from build123d import *

# Parameters (mm, degrees)
BOSS_EXTRUDE1_DEPTH = 6.5
SCALE1_SCALE        = 0.85
SKETCH2_R           = 9
CUT_EXTRUDE1_DEPTH  = 10
SKETCH7_R           = 2.1
CUT_EXTRUDE7_DEPTH  = 6
SKETCH8_R           = 2.1
CUT_EXTRUDE8_DEPTH  = 6
SKETCH9_R           = 2.1
CUT_EXTRUDE9_DEPTH  = 6
SKETCH10_R          = 2.1
CUT_EXTRUDE10_DEPTH = 10
SKETCH12_R          = 2.1
SKETCH12_R_2        = 9
BOSS_EXTRUDE2_DEPTH = 0.5
SKETCH13_R          = 2.1
SKETCH13_R_2        = 9
BOSS_EXTRUDE3_DEPTH = 0.5


with BuildPart() as part:
    # Sketch1 → Boss-Extrude1 (new body)
    with BuildSketch(Plane(origin=(0, 0, 0), x_dir=(1, 0, 0), z_dir=(0, 1, 0))):
        Polygon((1.965722873, 0), (57.111381005, 0), (70.055583492, 27.758931813), (45.577412376, 71.918721468), (13.499691502, 71.918721468), (-10.978479614, 27.758931813), align=None)
    extrude(amount=BOSS_EXTRUDE1_DEPTH)


with BuildPart() as part_1:
    # Scale1: scaled about (29.538551939, 3.25, -32.913795141)
    add(part.part.scale(SCALE1_SCALE).moved(Location((4.430782791, 0.4875, -4.937069271))))

    # Sketch2 → Cut-Extrude1 (cut)
    with BuildSketch(Plane(origin=(0, 6.0125, 0), x_dir=(1, 0, 0), z_dir=(0, 1, 0))):
        with Locations((29.561028759, 35.307348014)):
            Circle(SKETCH2_R)
    extrude(amount=-CUT_EXTRUDE1_DEPTH, mode=Mode.SUBTRACT)

    # Sketch7 → Cut-Extrude7 (cut)
    with BuildSketch(Plane(origin=(6.902862477, 0, -3.218857636), x_dir=(0.422618262, 0, 0.906307787), z_dir=(-0.906307787, 0, 0.422618262))):
        with Locations((-23.930140333, 3.2525)):
            Circle(SKETCH7_R)
        with Locations((-5.895836778, 3.2525)):
            Circle(SKETCH7_R)
    extrude(amount=-CUT_EXTRUDE7_DEPTH, mode=Mode.SUBTRACT)

    # Sketch8 → Cut-Extrude8 (cut)
    with BuildSketch(Plane(origin=(0, 0, -66.067982519), x_dir=(-1, 0, 0), z_dir=(0, 0, -1))):
        with Locations((-39.17158331, 3.2525)):
            Circle(SKETCH8_R)
        with Locations((-19.905520568, 3.2525)):
            Circle(SKETCH8_R)
    extrude(amount=-CUT_EXTRUDE8_DEPTH, mode=Mode.SUBTRACT)

    # Sketch9 → Cut-Extrude9 (cut)
    with BuildSketch(Plane(origin=(41.622704657, 0, 19.408985935), x_dir=(0.422618262, 0, -0.906307787), z_dir=(0.906307787, 0, 0.422618262))):
        with Locations((30.862899728, 3.2525)):
            Circle(SKETCH9_R)
        with Locations((48.897203282, 3.2525)):
            Circle(SKETCH9_R)
    extrude(amount=-CUT_EXTRUDE9_DEPTH, mode=Mode.SUBTRACT)

    # Sketch10 → Cut-Extrude10 (cut)
    with BuildSketch(Plane.XZ.offset(-0.4875)):
        with Locations((41.211489709, -54.443494734)):
            Circle(SKETCH10_R)
        with Locations((52.846920595, -33.452621763)):
            Circle(SKETCH10_R)
        with Locations((17.41315777, -53.627241783)):
            Circle(SKETCH10_R)
        with Locations((5.777726884, -32.636368812)):
            Circle(SKETCH10_R)
        with Locations((17.101647233, -12.287069271)):
            Circle(SKETCH10_R)
        with Locations((41.101647233, -12.287069271)):
            Circle(SKETCH10_R)
    extrude(amount=-CUT_EXTRUDE10_DEPTH, mode=Mode.SUBTRACT)

    # Sketch12 → Boss-Extrude2 (add)
    with BuildSketch(Plane(origin=(0, 6.0125, 0), x_dir=(1, 0, 0), z_dir=(0, 1, 0))):
        Polygon((-4.900924881, 28.532161313), (6.101647233, 4.937069271), (52.975456645, 4.937069271), (63.978028759, 28.532161313), (43.17158331, 66.067982519), (15.905520568, 66.067982519), align=None)
        with Locations((17.101647233, 12.287069271)):
            Circle(SKETCH12_R, mode=Mode.SUBTRACT)
        with Locations((41.211489709, 54.443494734)):
            Circle(SKETCH12_R, mode=Mode.SUBTRACT)
        with Locations((29.561028759, 35.307348014)):
            Circle(SKETCH12_R_2, mode=Mode.SUBTRACT)
        with Locations((5.777726884, 32.636368812)):
            Circle(SKETCH12_R, mode=Mode.SUBTRACT)
        with Locations((41.101647233, 12.287069271)):
            Circle(SKETCH12_R, mode=Mode.SUBTRACT)
        with Locations((52.846920595, 33.452621763)):
            Circle(SKETCH12_R, mode=Mode.SUBTRACT)
        with Locations((17.41315777, 53.627241783)):
            Circle(SKETCH12_R, mode=Mode.SUBTRACT)
    extrude(amount=BOSS_EXTRUDE2_DEPTH)

    # Sketch13 → Boss-Extrude3 (add)
    with BuildSketch(Plane.XZ.offset(-0.4875)):
        Polygon((6.101647233, -4.937069271), (-4.900924881, -28.532161313), (15.905520568, -66.067982519), (43.17158331, -66.067982519), (63.978028759, -28.532161313), (52.975456645, -4.937069271), align=None)
        with Locations((41.101647233, -12.287069271)):
            Circle(SKETCH13_R, mode=Mode.SUBTRACT)
        with Locations((17.101647233, -12.287069271)):
            Circle(SKETCH13_R, mode=Mode.SUBTRACT)
        with Locations((5.777726884, -32.636368812)):
            Circle(SKETCH13_R, mode=Mode.SUBTRACT)
        with Locations((41.211489709, -54.443494734)):
            Circle(SKETCH13_R, mode=Mode.SUBTRACT)
        with Locations((29.561028759, -35.307348014)):
            Circle(SKETCH13_R_2, mode=Mode.SUBTRACT)
        with Locations((52.846920595, -33.452621763)):
            Circle(SKETCH13_R, mode=Mode.SUBTRACT)
        with Locations((17.41315777, -53.627241783)):
            Circle(SKETCH13_R, mode=Mode.SUBTRACT)
    extrude(amount=BOSS_EXTRUDE3_DEPTH)


solid = part_1.part
Read the model definition and answer for the solid it produces. Units are mm, in the model's axes. A direction names the side the tool comes from. Give positions to 0.01 mm unless a question says otherwise; leave off trailing zeros. Write each loop counter-clockwise with the first axis right and the second up, starting at its lowest first coordinate (ties: lowest second). Pieces come first, ordered by that corner, then holes. Notation, with made-up numbers: (86, -27) - (92, -27) arc R23 cw to (92, 0) - close; hole circle Ø4 at (34.5, 13.25). An arc over 180 degrees is marked (long way). Answer in a Markdown table with one row per item. Add a question column.
Item 1: Determine the mould class of faces 4 (the face through (37, 6.512, -29)), 5 (the face through (56.84, 3.28, -27.42)) for opening direction X: pulls with the +X half, pulls with the -X half, needs draft (parallel to the pull), parting line crosses it, or undercut.
Item 2: Section A-A, the plane x = 31 is taken. Write down the section's boundary in (y, z), and give its area (3 significant figures).
Item 3: Section C-C, the plane x = 13 is taken. Write down the section's boundary in (y, z).
Item 4: Section D-D, the plane y = 2 is taken. Count the separate pieces of the cut face and the enclosed holes in it, and give its area (3 significant figures).
Item 5: Find the intervals of material crossed by L1, parallel to X at y = 4.5, z = -28; L2, parallel to X at y = 3, z = -32.5; L3, parallel to Z at x = 29, y = 6, in increasing order.
Item 6: Flat-ended cylindrical pins translate along their axes: P1, Ø2.5, axis at x = 52.85, z = -33.45, coming from the -Y side; P2, Ø1, axis at y = 5, z = -13.5, coming from the +X side; P3, Ø1.3, axis at x = 19.5, y = 3.5, coming from the -Z side. Find the tip coordinate at first contact, or state that the pin passes through.
Item 7: Section B-B, the plane z = -46 is taken. Write down the section's boundary in (x, y).
Item 8: A tool of negligible diameter and unlimited length cuts with its end or side. For faces 1 (the face through (17.9, 3.88, -63.11)), 2 (the face through (2.2, 3.3, -27.5)), 3 (the face through (30, 3, -4.937)), from which of +Z, -Z, +X, -X, +Y, -Y can it reach the whole face along a straight path? Write none if from no direction.
Recorded:
| question | item | result |
|---|---|---|
| 1 | face 4 | needs draft |
| 1 | face 5 | undercut |
| 2 | outline | (-0.01, -66.07) - (6.51, -66.07) - (6.51, -44.19) - (-0.01, -44.19) - close; (-0.01, -26.42) - (6.51, -26.42) - (6.51, -4.94) - (-0.01, -4.94) - close |
| 2 | area | 283 mm2 |
| 3 | outline | (-0.01, -60.83) - (6.51, -60.83) - (6.51, -4.94) - (-0.01, -4.94) - close |
| 4 | separate pieces | 1 |
| 4 | enclosed holes | 7 |
| 4 | area | 2,710 mm2 |
| 5 | L1 | x = -4.65 to -0.57, 1.97 to 24.31, 34.81 to 57.11, 59.65 to 63.73 |
| 5 | L2 | x = -2.7 to 3.68, 7.87 to 21.01, 38.11 to 50.98, 54.72 to 61.78 |
| 5 | L3 | z = -66.07 to -44.29, -26.32 to -4.94 |
| 6 | P1 | passes through |
| 6 | P2 | stops at x = 57.2 |
| 6 | P3 | stops at z = -60.07 |
| 7 | outline | (4.78, -0.01) - (54.3, -0.01) - (54.3, 6.51) - (4.78, 6.51) - close |
| 8 | face 1 | -Z |
| 8 | face 2 | none |
| 8 | face 3 | +Z, +X, -X, +Y, -Y |
